Part model, mm, in its own coordinate system. A direction names the side the tool comes from. Round coordinates to 2 decimals unless told otherwise and drop trailing zeros. Order: outer loops, then holes, each group sorted by start corner. A loop starts at its lowest first (then second) coordinate and runs counter-clockwise, first axis right, second up. Notation, with made-up numbers: (59.25, 19) - (99.25, 19) arc R28 ccw to (99.25, 40) - close; hole circle Ø10 at (-30.75, -38). An arc over 180 degrees is marked (long way). Answer as a JSON object with one key per item and string values.
```python
from build123d import *

# Parameters (mm, degrees)
F0_W     = 3.5
F0_H     = 16.5
F0_H_2   = 3.5
F0_W_2   = 16.5
F1_DEPTH = 15
F2_R     = 1.65
F4_DEPTH = 3.5
F2_R_2   = 2.75
F5_DEPTH = 1
F3_R     = 1.65
F6_DEPTH = 3.5
F3_R_2   = 2.75
F7_DEPTH = 1


with BuildPart() as f1:
    # F0 (on Top) → F1 (new body)
    with BuildSketch(Plane.XY):
        with Locations((-10.361038, 3.047789)):
            Rectangle(F0_W, F0_H)
        with Locations((-10.361038, -6.952211)):
            Rectangle(F0_W, F0_H_2)
        with Locations((-0.361038, -6.952211)):
            Rectangle(F0_W_2, F0_H_2)
    extrude(amount=F1_DEPTH)

    # F2 (on face) → F4 (cut, through all)
    with BuildSketch(Plane.YZ.offset(-8.611038)):
        with Locations((3.047789, 7.5)):
            Circle(F2_R)
    extrude(amount=-F4_DEPTH, mode=Mode.SUBTRACT)

    # F2 (on face) → F5 (cut)
    with BuildSketch(Plane.YZ.offset(-8.611038)):
        with Locations((3.047789, 7.5)):
            Circle(F2_R_2)
        with Locations((3.047789, 7.5)):
            Circle(F2_R, mode=Mode.SUBTRACT)
    extrude(amount=-F5_DEPTH, mode=Mode.SUBTRACT)

    # F3 (on face) → F6 (cut, through all)
    with BuildSketch(Plane(origin=(0, -5.202211, 0), x_dir=(-1, 0, 0), z_dir=(0, 1, 0))):
        with Locations((0.361038, 7.5)):
            Circle(F3_R)
    extrude(amount=-F6_DEPTH, mode=Mode.SUBTRACT)

    # F3 (on face) → F7 (cut)
    with BuildSketch(Plane(origin=(0, -5.202211, 0), x_dir=(-1, 0, 0), z_dir=(0, 1, 0))):
        with Locations((0.361038, 7.5)):
            Circle(F3_R_2)
        with Locations((0.361038, 7.5)):
            Circle(F3_R, mode=Mode.SUBTRACT)
    extrude(amount=-F7_DEPTH, mode=Mode.SUBTRACT)


solid = f1.part
```
Item 1: Probe L1, parallel to Y at x = -2.5, z = 9; L2, parallel to Y at x = -4.25, z = 2.25; L3, parallel to X at y = -5.25, z = 8.25. List the from-to ranges inside material, lowest first. Write a range as from..to.
Taken from the geometry:
{"L1": "-8.7..-6.2", "L2": "-8.7..-5.2", "L3": "-12.11..-3.01, 2.28..7.89"}
Item 2: Cut at D-D (y = -0.25). Write the cut outline in (x, z).
Taken from the geometry:
{"outline": "(-12.11, 0) - (-8.61, 0) - (-8.61, 15) - (-12.11, 15) - close"}
Item 3: Tool access for faces 5 (the flat face through (-9.611, 3, 5.7)), 6 (the flat face through (-2, -6.202, 6)), 7 (the flat face through (-8.611, 3, 4)): list every direction of +Z, -Z, +X, -X, +Y, -Y with a clear straight run to the whole face (end or side of a thin tool).
Taken from the geometry:
{"face 5": "+X", "face 6": "+Y", "face 7": "+Z, -Z, +X, +Y"}
Item 4: Two-plate mould, pull along Z, no slides. Class faces 1 (the flat face through (-9, -3, 0)), 2 (the cylindrical face through (0.235, -5.695, 4.815)), 3 (the flat face through (0, -5.202, 4)), 4 (the cylindrical face through (-9.1, 4.32, 5.06)): pulls with the +Z half, pulls with the -Z half, needs draft (parallel to the pull), parting line crosses it, or undercut.
Taken from the geometry:
{"face 1": "pulls with the -Z half", "face 2": "undercut", "face 3": "needs draft", "face 4": "undercut"}
Item 5: Cut at C-C (x = -2.5). Write the cut outline in (y, z), plus the area to 3 significant figures.
Taken from the geometry:
{"outline": "(-8.7, 0) - (-5.2, 0) - (-5.2, 5.77) - (-6.2, 5.77) - (-6.2, 9.23) - (-5.2, 9.23) - (-5.2, 15) - (-8.7, 15) - close", "area": "49.0 mm2"}
Item 6: Cut at B-B (y = 3). Write the cut outline in (x, z).
Taken from the geometry:
{"outline": "(-12.11, 0) - (-8.61, 0) - (-8.61, 4.75) - (-9.61, 4.75) - (-9.61, 5.85) - (-12.11, 5.85) - close; (-12.11, 9.15) - (-9.61, 9.15) - (-9.61, 10.25) - (-8.61, 10.25) - (-8.61, 15) - (-12.11, 15) - close"}
Item 7: Drop flat-ended pins along their axis: P1, Ø6, axis at x = -1.5, z = 7.5, coming from the +Y side; P2, Ø7.5, axis at y = 5.5, z = 5, coming from the +X side; P3, Ø5, axis at y = 3.05, z = 7.5, coming from the +X side. Give the stop position or say it passes through.
Taken from the geometry:
{"P1": "y = -5.2", "P2": "x = -8.61", "P3": "x = -9.61"}
Item 8: Cut at A-A (z = 7.5). Write the cut outline in (x, y), plus the area to 3 significant figures.
Taken from the geometry:
{"outline": "(-12.11, -8.7) - (-2.01, -8.7) - (-2.01, -6.2) - (-3.11, -6.2) - (-3.11, -5.2) - (-8.61, -5.2) - (-8.61, 0.3) - (-9.61, 0.3) - (-9.61, 1.4) - (-12.11, 1.4) - close; (-12.11, 4.7) - (-9.61, 4.7) - (-9.61, 5.8) - (-8.61, 5.8) - (-8.61, 11.3) - (-12.11, 11.3) - close; (1.29, -8.7) - (7.89, -8.7) - (7.89, -5.2) - (2.39, -5.2) - (2.39, -6.2) - (1.29, -6.2) - close", "area": "100 mm2"}
